The figure shows three views and two pictorial views of one solid part (mm, origin at its lowest corner). Answer the questions. Coordinates: 2 decimals unless noted, no trailing zeros. Order: outer loops, then holes, each group sorted by start corner. A loop starts at its lowest first (then second) coordinate and runs counter-clockwise, first axis right, second up.
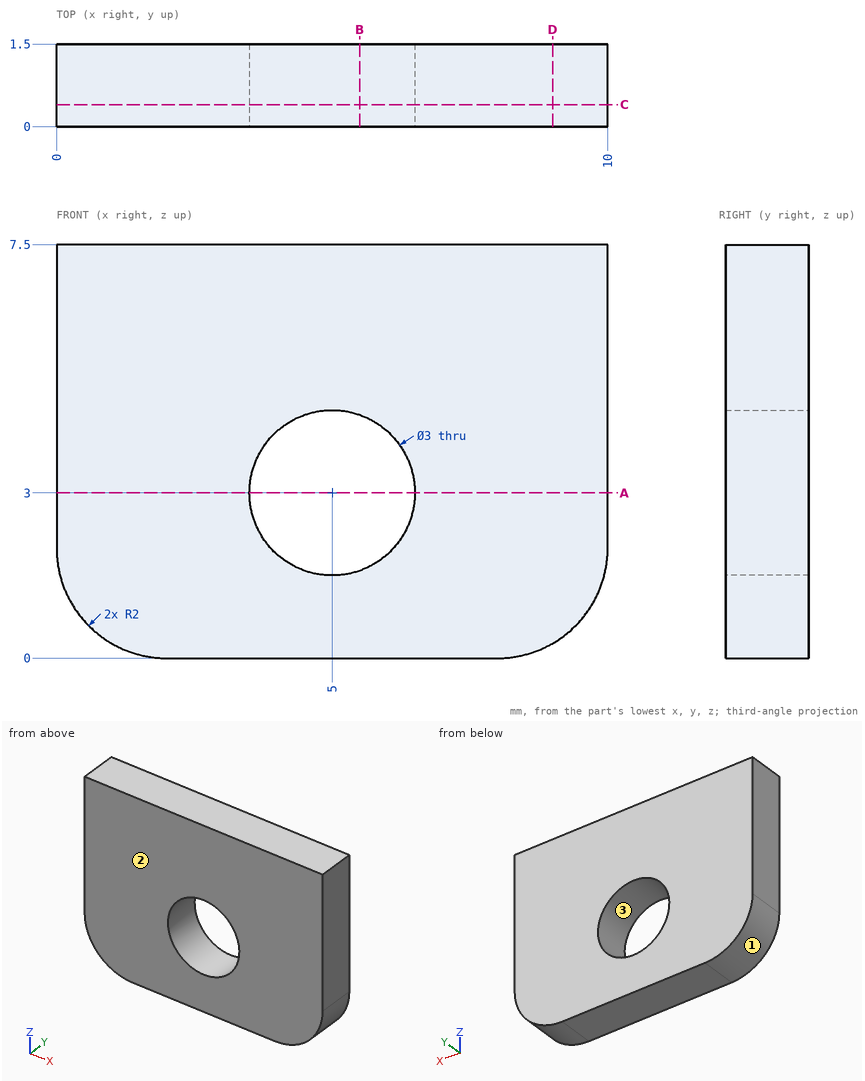
Q1. Determine the mould class of the marked faces 1, 2 and 3 for opening direction X: +X half, -X half, draft (parallel to the pull), parting line (faces both ways), or undercut.
Q2. This flat-tipped pin is pushed along its axis until it touches: P1, Ø1.8, axis at x = 5, z = 3, coming from the -Y side. Where does it stop, or does it pass through?
Q3. The part is cut by section C-C, the plane y = 0.4. Determine the outline of the cut face in (x, z).
Q4. The part is cut by section D-D, the plane x = 9. Determine the outline of the cut face in (y, z), then the cut area to 3 significant figures.
Q5. The part is cut by section A-A, the plane z = 3. Determine the outline of the cut face in (x, y).
Q6. Straight lines are drawn through the part: L1, parallel to X at y = 0.8, z = 3; L2, parallel to Z at x = 6.25, y = 1.45; L3, parallel to Z at x = 4.25, y = 0.65. For each, find the intervals that lie inside material, in ascending order.
Q7. The part is cut by section B-B, the plane x = 5.5. Determine the outline of the cut face in (y, z), then the cut area to 3 significant figures.
Computed values:
1. face 1: -X half
1. face 2: draft
1. face 3: undercut
2. P1: passes through
3. outline: (0, 2) arc R2 ccw to (2, 0) - (8, 0) arc R2 ccw to (10, 2) - (10, 7.5) - (0, 7.5) - close; hole circle Ø3 at (5, 3)
4. outline: (0, 0.27) - (1.5, 0.27) - (1.5, 7.5) - (0, 7.5) - close
4. area: 10.8 mm2
5. outline: (0, 0) - (3.5, 0) - (3.5, 1.5) - (0, 1.5) - close; (6.5, 0) - (10, 0) - (10, 1.5) - (6.5, 1.5) - close
6. L1: x = 0 to 3.5, 6.5 to 10
6. L2: z = 0 to 2.17, 3.83 to 7.5
6. L3: z = 0 to 1.7, 4.3 to 7.5
7. outline: (0, 0) - (1.5, 0) - (1.5, 1.59) - (0, 1.59) - close; (0, 4.41) - (1.5, 4.41) - (1.5, 7.5) - (0, 7.5) - close
7. area: 7.01 mm2
